```python
from build123d import *

# Parameters (mm, degrees)
SKETCH1_R           = 2.499995
BOSS_EXTRUDE1_DEPTH = 3.175


with BuildPart() as part:
    # Sketch1 → Boss-Extrude1 (new body)
    with BuildSketch(Plane(origin=(0, 0, 0), x_dir=(1, 0, 0), z_dir=(0, 1, 0))):
        with BuildLine():
            Line((-13.993314597, 28.4999938), (-25.9599938, 28.4999938))
            ThreePointArc((-25.9599938, 28.4999938), (-27.756045024, 27.756045024), (-28.4999938, 25.9599938))
            Line((-28.4999938, 25.9599938), (-28.4999938, 13.993314597))
            Line((-28.4999938, 13.993314597), (-28.4999938, -13.993314597))
            Line((-28.4999938, -13.993314597), (-28.4999938, -25.9599938))
            ThreePointArc((-28.4999938, -25.9599938), (-27.756045024, -27.756045024), (-25.9599938, -28.4999938))
            Line((-25.9599938, -28.4999938), (-13.993314597, -28.4999938))
            Line((-13.993314597, -28.4999938), (13.993314597, -28.4999938))
            Line((13.993314597, -28.4999938), (25.9599938, -28.4999938))
            ThreePointArc((25.9599938, -28.4999938), (27.756045024, -27.756045024), (28.4999938, -25.9599938))
            Line((28.4999938, -25.9599938), (28.4999938, -13.993314597))
            Line((28.4999938, -13.993314597), (28.4999938, 13.993314597))
            Line((28.4999938, 13.993314597), (28.4999938, 25.9599938))
            ThreePointArc((28.4999938, 25.9599938), (27.756045024, 27.756045024), (25.9599938, 28.4999938))
            Line((25.9599938, 28.4999938), (13.993314597, 28.4999938))
            Line((13.993314597, 28.4999938), (-13.993314597, 28.4999938))
        make_face()
        with Locations((-23.5000038, 23.5000038)):
            Circle(SKETCH1_R, mode=Mode.SUBTRACT)
        with Locations((23.5000038, 23.5000038)):
            Circle(SKETCH1_R, mode=Mode.SUBTRACT)
        with Locations((23.5000038, -23.5000038)):
            Circle(SKETCH1_R, mode=Mode.SUBTRACT)
        with Locations((-23.5000038, -23.5000038)):
            Circle(SKETCH1_R, mode=Mode.SUBTRACT)
        with BuildLine():
            Line((17.525786369, -21.990248683), (15.587608536, -20.05458701))
            ThreePointArc((15.587608536, -20.05458701), (0.016497958, -25.399994642), (-15.561543442, -20.074819195))
            Line((-15.561543442, -20.074819195), (-17.497205115, -22.012997028))
            Line((-17.497205115, -22.012997028), (-21.990248683, -17.525786369))
            Line((-21.990248683, -17.525786369), (-20.05458701, -15.587608536))
            ThreePointArc((-20.05458701, -15.587608536), (-25.399994642, -0.016497958), (-20.074819195, 15.561543442))
            Line((-20.074819195, 15.561543442), (-22.012997028, 17.497205115))
            Line((-22.012997028, 17.497205115), (-17.525786369, 21.990248683))
            Line((-17.525786369, 21.990248683), (-15.587608536, 20.05458701))
            ThreePointArc((-15.587608536, 20.05458701), (-0.016497958, 25.399994642), (15.561543442, 20.074819195))
            Line((15.561543442, 20.074819195), (17.497205115, 22.012997028))
            Line((17.497205115, 22.012997028), (21.990248683, 17.525786369))
            Line((21.990248683, 17.525786369), (20.05458701, 15.587608536))
            ThreePointArc((20.05458701, 15.587608536), (25.399994642, 0.016497958), (20.074819195, -15.561543442))
            Line((20.074819195, -15.561543442), (22.012997028, -17.497205115))
            Line((22.012997028, -17.497205115), (17.525786369, -21.990248683))
        make_face(mode=Mode.SUBTRACT)
    extrude(amount=BOSS_EXTRUDE1_DEPTH)


solid = part.part
```
Read the model definition and answer for the solid it produces. Units are mm, in the model's axes. A direction names the side the tool comes from. Give positions to 0.01 mm unless a question says otherwise; leave off trailing zeros. Write each loop counter-clockwise with the first axis right and the second up, starting at its lowest first coordinate (ties: lowest second). Pieces come first, ordered by that corner, then holes. Notation, with made-up numbers: (13, 67.5) -> (71, 67.5) arc R28 ccw to (71, 90.5) -> close; hole circle Ø11 at (87, -24.75). An arc over 180 degrees is marked (long way). Answer as a JSON object with one key per item and string values.
1) For a pull along X with two mould halves and no side action, classify faces 3 (the flat face through (19.712, 1.565, -19.801)), 4 (the cylindrical face through (0.3, 1.6, 25.4)), 5 (the cylindrical face through (-27.736, 1.565, -27.776)), 6 (the flat face through (28.5, 2, 0)) as pulls with the +X half, pulls with the -X half, needs draft (parallel to the pull), parting line crosses it, or undercut.
Findings below:
{"face 3": "undercut", "face 4": "undercut", "face 5": "pulls with the -X half", "face 6": "pulls with the +X half"}
2) Straight lines are drawn through the part: probe 1 along Z at (x, y) = (25.5, 2.85); probe 2 along X at (y, z) = (1.2, 0.5); probe 3 along Z at (x, y) = (18.5, 1.6). For each, find the intervals that lie inside material, in ascending order. Write a range as from..to.
Findings below:
{"probe 1": "z = -28.5..-25, -22..22, 25..28.5", "probe 2": "x = -28.5..-25.4, 25.4..28.5", "probe 3": "z = -28.5..-21.01, 21.01..28.5"}
3) Section B-B on z = 3.5 is taken. Write down the section's boundary in (x, y) (3 decimals).
Findings below:
{"outline": "(-28.5, 0) -> (-25.158, 0) -> (-25.158, 3.175) -> (-28.5, 3.175) -> close; (25.158, 0) -> (28.5, 0) -> (28.5, 3.175) -> (25.158, 3.175) -> close"}
4) A flat-ended cylindrical pin translates along its axis: pin 1 Ø12 at (x, z) = (3, 19.5) entering from -Y. Find the tip coordinate at first contact, or state that the pin passes through.
Findings below:
{"pin 1": "stops at y = 0"}
5) Section A-A on x = -5 is taken. Write down the section's boundary in (y, z) (3 decimals), then the cut area to 3 significant figures.
Findings below:
{"outline": "(0, -28.5) -> (3.175, -28.5) -> (3.175, -24.903) -> (0, -24.903) -> close; (0, 24.903) -> (3.175, 24.903) -> (3.175, 28.5) -> (0, 28.5) -> close", "area": "22.8 mm^2"}
6) Section C-C on y = 0.8 is taken. Write down the section's boundary in (x, z), then the cut area to 3 significant figures.
Findings below:
{"outline": "(-28.5, -25.96) arc R2.54 ccw to (-25.96, -28.5) -> (25.96, -28.5) arc R2.54 ccw to (28.5, -25.96) -> (28.5, 25.96) arc R2.54 ccw to (25.96, 28.5) -> (-25.96, 28.5) arc R2.54 ccw to (-28.5, 25.96) -> close; hole circle Ø5 at (-23.5, -23.5); hole circle Ø5 at (-23.5, 23.5); hole (-22.01, -17.5) -> (-17.53, -21.99) -> (-15.59, -20.05) arc R25.4 ccw to (15.56, -20.07) -> (17.5, -22.01) -> (21.99, -17.53) -> (20.05, -15.59) arc R25.4 ccw to (20.07, 15.56) -> (22.01, 17.5) -> (17.53, 21.99) -> (15.59, 20.05) arc R25.4 ccw to (-15.56, 20.07) -> (-17.5, 22.01) -> (-21.99, 17.53) -> (-20.05, 15.59) arc R25.4 ccw to (-20.07, -15.56) -> close; hole circle Ø5 at (23.5, -23.5); hole circle Ø5 at (23.5, 23.5)", "area": "1,070 mm^2"}
7) A tool of negligible diameter and unlimited length cuts with its end or side. For faces 1 (the flat face through (16.57, 1.565, 21.036)), 2 (the flat face through (0, 2, -28.5)), from which of +Z, -Z, +X, -X, +Y, -Y can it reach the whole face along a straight path? Write none if from no direction.
Findings below:
{"face 1": "+Y, -Y", "face 2": "-Z, +X, -X, +Y, -Y"}
